The model under review builds one solid part; all positions refer to its coordinate system, in mm. A direction names the side the tool comes from. Round coordinates to 2 decimals unless told otherwise and drop trailing zeros. Loops run counter-clockwise (first coordinate to the right, second up) from the corner with the lowest first, then second, coordinate; pieces in that order, holes last. Notation, with made-up numbers: M -40,55 L -19,55 A21 ccw -19,88 Z; hole C 47.25,75.25 d11. An arc over 180 degrees is marked long. One line per question, with ' | ' between items.
from build123d import *

# Parameters (mm, degrees)
F0_R        = 28.9544209137
F0_R_2      = 21.0693
F1_DEPTH    = 152.4
F2_R        = 31.75
F3_DEPTH    = 19.05
F4_W        = 39.7148355842
F4_H        = 16.8466605246
F5_DEPTH    = 38.1
F6_R        = 9.2348971927
F7_DEPTH    = 25.4
F8_T1_DEPTH = 118.4466605246
F9_R        = 2.54


# Not quite as in the source:
# - a fillet or chamfer that OpenCascade refuses, or shapes differently, is made with other operations: its cross-section is extruded or revolved along the edge and cut away or added


with BuildPart() as f1:
    # F0 (on Top) → F1 (new body)
    with BuildSketch(Plane.XY):
        Circle(F0_R)
        Circle(F0_R_2, mode=Mode.SUBTRACT)
    extrude(amount=F1_DEPTH)

    # F2 (on face) → F3 (join)
    with BuildSketch(Plane.XY.offset(152.4)):
        Circle(F2_R)
    extrude(amount=F3_DEPTH)

    # F4 (on face) → F5 (join)
    with BuildSketch(Plane.XY.offset(171.45)):
        Rectangle(F4_W, F4_H)
    extrude(amount=F5_DEPTH)

    # F6 (on face) → F7 (cut)
    with BuildSketch(Plane.XZ.offset(8.4233302623)):
        with Locations((0, 190.5)):
            Circle(F6_R)
    extrude(amount=-F7_DEPTH, mode=Mode.SUBTRACT)

    # F8: fillet of radius 20.32 on 2 edges, made by hand

    # F8_s2 → F8_t1 (cut)
    with BuildSketch(Plane.XZ.offset(-59.2233302623)):
        with BuildLine():
            ThreePointArc((19.8574177921, 189.23), (13.9058275858, 203.5984097937), (-0.4625822079, 209.55))
            Line((-0.4625822079, 209.55), (19.8574177921, 209.55))
            Line((19.8574177921, 209.55), (19.8574177921, 189.23))
        make_face()
        with BuildLine():
            ThreePointArc((-19.8574177921, 189.23), (-13.9058275858, 203.5984097937), (0.4625822079, 209.55))
            Line((0.4625822079, 209.55), (-19.8574177921, 209.55))
            Line((-19.8574177921, 209.55), (-19.8574177921, 189.23))
        make_face()
    extrude(amount=F8_T1_DEPTH, mode=Mode.SUBTRACT)

    # F9
    f9_edges = [f1.edges().sort_by_distance(p)[0] for p in [
        (19.857418, -8.42333, 180.34),
        (14.068455, -8.42333, 203.433921),
        (-14.068455, -8.42333, 203.433921),
        (-19.857418, -8.42333, 180.34),
        (0, -8.42333, 171.45),
        (19.857418, 0, 171.45),
        (-28.954421, 0, 152.4),
        (-21.0693, 0, 152.4),
        (19.857418, 8.42333, 180.34),
        (14.068455, 8.42333, 203.433921),
        (-14.068455, 8.42333, 203.433921),
        (0, 8.42333, 171.45),
        (-19.857418, 0, 171.45),
        (-19.857418, 8.42333, 180.34),
    ]]
    fillet(f9_edges, radius=F9_R)


solid = f1.part
1) Mouldability with a two-part tool opening along X and no side actions: class faces 5 (the cylindrical face through (9.722, -18.692, 73.881)), 6 (the flat face through (0, 0, 152.4)), 7 (the flat face through (-19.857, 0, 182)), 8 (the cylindrical face through (26.747, -11.09, 73.881)) as +X half, -X half, draft (parallel to the pull), parting line (faces both ways), or undercut.
Output values:
face 5: undercut | face 6: undercut | face 7: -X half | face 8: parting line
2) Add section B-B on z = 85. State the section outline as (x, y) points.
Output values:
outline: C 0,0 d57.91; hole C 0,0 d42.14
3) Add section C-C on z = 155. State the section outline as (x, y) points.
Output values:
outline: C 0,0 d63.5
4) Machinability: for faces 1 (the flat face through (7, 8.423, 183)), 2 (the flat face through (7, -8.423, 183)), 3 (the flat face through (19.857, 0, 182)), 4 (the cylindrical face through (-6.883, -30.995, 161.792)), which of the approach directions +Z, -Z, +X, -X, +Y, -Y give a long, thin tool a straight path to every point of the face, cutting with its end or side? Answer none if there is none.
Output values:
face 1: +Z, +X, -X, +Y | face 2: +Z, +X, -X, -Y | face 3: +Z, +X, +Y, -Y | face 4: +Z, -Z
5) For line 1 (Y direction, x = 0, z = 89.5); line 2 (X direction, y = -15, z = 146); line 3 (Z direction, x = -6.5, y = 10.5), list the stretches that pass through material, from the lowest coordinate up.
Output values:
line 1: y = -28.95 to -21.07, 21.07 to 28.95 | line 2: x = -24.77 to -14.8, 14.8 to 24.77 | line 3: z = 152.4 to 171.49
6) Insertion check: P1, Ø3, axis at x = -12.5, y = 4, coming from the -Z side; P2, Ø13, axis at y = 1, z = 182, coming from the +X side; P3, Ø6, axis at y = 1.5, z = 181, coming from the -X side; P4, Ø11, axis at x = 0, z = 190.5, coming from the +Y side. Each pin has a flat end and moves straight along its axis. Give the tip position at first contact, or say it passes through.
Output values:
P1: stops at z = 152.4 | P2: stops at x = 19.86 | P3: stops at x = -19.86 | P4: passes through
7) Add section A-A on y = 0. State the section outline as (x, z) points, then the cut area to 3 significant figures.
Output values:
outline: M -31.75,152.4 L -31.49,152.4 A2.54 cw -28.95,149.86 L -28.95,0 L -21.07,0 L -21.07,149.86 A2.54 cw -18.53,152.4 L 18.53,152.4 A2.54 cw 21.07,149.86 L 21.07,0 L 28.95,0 L 28.95,149.86 A2.54 cw 31.49,152.4 L 31.75,152.4 L 31.75,171.45 L 22.4,171.45 A2.54 cw 19.86,173.99 L 19.86,189.23 A20.32 ccw 0,209.54 A20.32 ccw -19.86,189.23 L -19.86,173.99 A2.54 cw -22.4,171.45 L -31.75,171.45 Z; hole C 0,190.5 d18.47 | area: 4,690 mm²
